Could you check a few things on this model? Use its own coordinates, in mm. A direction names the side the tool comes from. Give positions to 0.01 mm unless a question says otherwise; leave off trailing zeros. Loops run counter-clockwise (first coordinate to the right, second up) from the corner with the lowest first, then second, coordinate; pieces in that order, holes last.
1. For P1, Ø3.5, axis at y = -1.5, z = -1, coming from the +X side; P2, Ø5, axis at x = 0.5, z = 1, coming from the +Y side; P3, Ø0.8, axis at x = 9.5, z = -5.5, coming from the +Y side, each with a flat end and sliding along its axis, tell me the tip position at first contact or that it passes through.
2. Imagine slicing it at A-A (y = 6.25). List the corners of the cut face in (x, z) for me.
3. Imagine slicing it at B-B (y = 4.5). List the corners of the cut face in (x, z) for me.
4. I need wall thicknesses on line 1 along X through (y, z) = (-1.5, -1); line 2 along Z through (x, y) = (10.1, 4.5); line 3 along X through (y, z) = (1, -5.25). Which ranges of each line are inside material? Lowest first, please.
5. For faces 1 (the flat face through (16, 3, -3.5)), 2 (the flat face through (0, 0, 0)), 3 (the cylindrical face through (8.75, 4.63, -5.01)), 4 (the flat face through (0.5, -1, 0)), 5 (the flat face through (15.5, 6, -6)), which set-ups out of +Z, -Z, +X, -X, +Y, -Y let a thin tool reach every point of the face, with its end or its side?
6. Imagine slicing it at C-C (z = -1.5). List the corners of the cut face in (x, y) for me.
7. Imagine slicing it at D-D (x = -6). List the corners of the cut face in (y, z) for me, plus the area to 3 significant figures.
8. Thinking about a two-plate mould opening in Z: for faces 6 (the flat face through (-6.5, -1, 0)), 7 (the flat face through (-3.5, -1, 0)), 8 (the flat face through (17, 13, -6)), 9 (the flat face through (0, -1, 8.5)), which applies, +Z half, -Z half, draft (parallel to the pull), parting line (faces both ways), or undercut?
```python
from build123d import *

# Parameters (mm, degrees)
F0_W      = 17
F0_H      = 17
F0_W_2    = 3
F0_H_2    = 13
F1_DEPTH  = 3
F2_W      = 3
F2_H      = 5
F3_DEPTH  = 10
F4_W      = 3
F4_H      = 5
F5_DEPTH  = 13
F6_W      = 2
F6_H      = 5
F7_DEPTH  = 7
F8_W      = 1
F8_H      = 5
F9_DEPTH  = 5
F10_R     = 1
F11_DEPTH = 3
F12_R     = 1.49999


# Not quite as in the source:
# - a fillet or chamfer is up to 0.001 mm smaller than in the source, because OpenCascade refuses the exact size


with BuildPart() as f1:
    # F0 (on Front) → F1 (new body)
    with BuildSketch(Plane.XZ):
        Rectangle(F0_W, F0_H)
        with Locations((-5, 0)):
            Rectangle(F0_W_2, F0_H_2, mode=Mode.SUBTRACT)
        with Locations((2, 0)):
            Rectangle(F0_W_2, F0_H_2, mode=Mode.SUBTRACT)
    extrude(amount=F1_DEPTH)

    # F2 (on face) → F3 (join)
    with BuildSketch(Plane.YZ.offset(8.5)):
        with Locations((-1.5, -6)):
            Rectangle(F2_W, F2_H)
    extrude(amount=F3_DEPTH)

    # F4 (on face) → F5 (join)
    with BuildSketch(Plane(origin=(0, 0, 0), x_dir=(-1, 0, 0), z_dir=(0, 1, 0))):
        with Locations((-17, -6)):
            Rectangle(F4_W, F4_H)
    extrude(amount=F5_DEPTH)

    # F6 (on face) → F7 (join)
    with BuildSketch(Plane(origin=(0, 0, 0), x_dir=(-1, 0, 0), z_dir=(0, 1, 0))):
        with Locations((-9.5, -6)):
            Rectangle(F6_W, F6_H)
    extrude(amount=F7_DEPTH)

    # F8 (on face) → F9 (cut)
    with BuildSketch(Plane(origin=(0, 7, 0), x_dir=(-1, 0, 0), z_dir=(0, 1, 0))):
        with Locations((-9.5, -6)):
            Rectangle(F8_W, F8_H)
    extrude(amount=-F9_DEPTH, mode=Mode.SUBTRACT)

    # F10 (on face) → F11 (cut)
    with BuildSketch(Plane(origin=(8.5, 0, 0), x_dir=(0, -1, 0), z_dir=(-1, 0, 0))):
        with Locations((-4.5, -6)):
            Circle(F10_R)
    extrude(amount=-F11_DEPTH, mode=Mode.SUBTRACT)

    # F12 (radius 1.5 in the source; OpenCascade refuses exactly that, so slightly less here)
    f12_edges = [f1.edges().sort_by_distance(p)[0] for p in [
        (-6.5, -1.5, 6.5),
        (0.5, -1.5, 6.5),
        (3.5, -1.5, 6.5),
        (-3.5, -1.5, 6.5),
        (-3.5, -1.5, -6.5),
        (3.5, -1.5, -6.5),
        (0.5, -1.5, -6.5),
        (-6.5, -1.5, -6.5),
    ]]
    fillet(f12_edges, radius=F12_R)


solid = f1.part
```
Derived:
1. P1: stops at x = 8.5
1. P2: stops at y = 0
1. P3: stops at y = 2
2. outline: (8.5, -8.5) - (9, -8.5) - (9, -3.5) - (8.5, -3.5) - close; (10, -8.5) - (10.5, -8.5) - (10.5, -3.5) - (10, -3.5) - close; (15.5, -8.5) - (18.5, -8.5) - (18.5, -3.5) - (15.5, -3.5) - close
3. outline: (8.5, -8.5) - (9, -8.5) - (9, -7) - (8.5, -7) - close; (8.5, -5) - (9, -5) - (9, -3.5) - (8.5, -3.5) - close; (10, -8.5) - (10.5, -8.5) - (10.5, -7) - (10, -7) - close; (10, -5) - (10.5, -5) - (10.5, -3.5) - (10, -3.5) - close; (15.5, -8.5) - (18.5, -8.5) - (18.5, -3.5) - (15.5, -3.5) - close
4. line 1: x = -8.5 to -6.5, -3.5 to 0.5, 3.5 to 8.5
4. line 2: z = -8.5 to -7, -5 to -3.5
4. line 3: x = 8.5 to 10.5, 15.5 to 18.5
5. face 1: +Z, +X, +Y, -Y
5. face 2: +Z, -Z, -X, +Y
5. face 3: -X
5. face 4: +Y, -Y
5. face 5: +Z, -Z, +Y
6. outline: (-8.5, -3) - (-6.5, -3) - (-6.5, 0) - (-8.5, 0) - close; (-3.5, -3) - (0.5, -3) - (0.5, 0) - (-3.5, 0) - close; (3.5, -3) - (8.5, -3) - (8.5, 0) - (3.5, 0) - close
7. outline: (-3, -8.5) - (0, -8.5) - (0, -6.12) - (-3, -6.12) - close; (-3, 6.12) - (0, 6.12) - (0, 8.5) - (-3, 8.5) - close
7. area: 14.3 mm2
8. face 6: undercut
8. face 7: undercut
8. face 8: draft
8. face 9: +Z half
